```python
from build123d import *

# Parameters (mm, degrees)
F0_W     = 20.4
F0_H     = 12.38
F1_DEPTH = 9.92
F3_D     = 9.7
F4_R     = 5.08
F5_W     = 1.75
F5_H     = 6.2
F6_DEPTH = 6
F7_R     = 5.08


with BuildPart() as f1:
    # F0 (on Front) → F1 (new body)
    with BuildSketch(Plane.XZ):
        Rectangle(F0_W, F0_H)
    extrude(amount=F1_DEPTH)

    # F3 (through all)
    with Locations(Plane.XZ.offset(9.92)):
        with Locations((0, 0)):
            Hole(F3_D / 2)

    # F4
    f4_edges = [f1.edges().sort_by_distance(p)[0] for p in [
        (10.2, -4.96, 6.19),
    ]]
    fillet(f4_edges, radius=F4_R)

    # F5 (on face) → F6 (cut)
    with BuildSketch(Plane.XY.offset(6.19)):
        with Locations((-7.325, -5.0558)):
            Rectangle(F5_W, F5_H)
    extrude(amount=-F6_DEPTH, mode=Mode.SUBTRACT)

    # F7
    f7_edges = [f1.edges().sort_by_distance(p)[0] for p in [
        (-10.2, -4.96, -6.19),
    ]]
    fillet(f7_edges, radius=F7_R)


solid = f1.part
```
Work out the finished part from the listing and answer in its coordinate system (mm). A direction names the side the tool comes from. Give positions to 0.01 mm unless a question says otherwise; leave off trailing zeros. Write each loop counter-clockwise with the first axis right and the second up, starting at its lowest first coordinate (ties: lowest second). Pieces come first, ordered by that corner, then holes.
(1) The part is cut by section B-B on y = -1.5. Write down the section's boundary in (x, z), plus the area to 3 significant figures.
Final values:
outline: (-10.2, -1.11) arc R5.08 ccw to (-5.12, -6.19) - (10.2, -6.19) - (10.2, 1.11) arc R5.08 ccw to (5.12, 6.19) - (-10.2, 6.19) - close; hole circle Ø9.7 at (0, 0)
area: 168 mm2
(2) The part is cut by section C-C on z = 2.5. Write down the section's boundary in (x, y), plus the area to 3 significant figures.
Final values:
outline: (-10.2, -9.92) - (-4.16, -9.92) - (-4.16, 0) - (-10.2, 0) - close; (4.16, -9.92) - (10.01, -9.92) - (10.01, 0) - (4.16, 0) - close; hole (-8.2, -8.16) - (-6.45, -8.16) - (-6.45, -1.96) - (-8.2, -1.96) - close
area: 107 mm2
(3) The part is cut by section A-A on x = 0. Write down the section's boundary in (y, z), plus the area to 3 significant figures.
Final values:
outline: (-9.92, -6.19) - (0, -6.19) - (0, -4.85) - (-9.92, -4.85) - close; (-9.92, 4.85) - (0, 4.85) - (0, 6.19) - (-9.92, 6.19) - close
area: 26.6 mm2
(4) The mould has two halves that part along X. Classify faces 1 (the flat face through (-8.2, -5, 3)), 2 (the cylindrical face through (8.672, -5.029, 4.741)), 3 (the flat face through (-5, 0, 1)): pulls with the +X half, pulls with the -X half, needs draft (parallel to the pull), parting line crosses it, or undercut.
Final values:
face 1: undercut
face 2: pulls with the +X half
face 3: needs draft
(5) A flat-ended cylindrical pin translates along its axis: pin 1 Ø3 at (y, z) = (-1.5, 3) entering from +X (3 decimals). Find the tip coordinate at first contact, or state that the pin passes through.
Final values:
pin 1: stops at x = 10.185
(6) The part is cut by section D-D on z = -4. Write down the section's boundary in (x, y).
Final values:
outline: (-9.3, -9.92) - (-2.74, -9.92) - (-2.74, 0) - (-9.3, 0) - close; (2.74, -9.92) - (10.2, -9.92) - (10.2, 0) - (2.74, 0) - close
(7) Which of the six approach directions +Z, -Z, +X, -X, +Y, -Y give full straight-line access (tool end or side, diameter ignored) to faces 4 (the flat face through (-7, -8.156, 3)), 5 (the flat face through (-5, -9.92, 1))?
Final values:
face 4: +Z
face 5: +Z, -Z, +X, -X, -Y
(8) Straight lines are drawn through the part: line 1 (Y direction, x = -6.75, z = 3.75); line 2 (X direction, y = -5.5, z = 1.5) (3 decimals); line 3 (Z direction, x = 0, y = -6.75). For each, find the intervals that lie inside material, in ascending order.
Final values:
line 1: y = -9.92 to -8.16, -1.96 to 0
line 2: x = -10.2 to -8.2, -6.45 to -4.612, 4.612 to 10.185
line 3: z = -6.19 to -4.85, 4.85 to 6.19
